Autodesk Inventor part; units mm, degrees
ref_plane "YZ Plane" through (0, 0, 0) normal (1, 0, 0) x (0, 1, 0)
ref_plane "XZ Plane" through (0, 0, 0) normal (0, 1, 0) x (-1, 0, 0)
ref_plane "XY Plane" through (0, 0, 0) normal (0, 0, 1) x (1, 0, 0)
sketch "Sketch1" plane through (0, 0, 0) normal (1, 0, 0) x (0, 1, 0)
  line L0 (31.75, 38.1) -> (6.35, 38.1)
  line L1 (6.35, 38.1) -> (6.35, -19.05)
  line L2 (6.35, -19.05) -> (31.75, -19.05)
  circle A0 centre (19.0246, 25.4) radius 3.175
  line L3 (0, 0) -> (6.35, 0)
  line L4 (0, 14.2875) -> (0, -6.35)
  circle A1 centre (19.05, -7.62) radius 3.175
  line L5 (31.75, 38.1) -> (31.75, -25.4)
  point P0 (31.75, -19.05)
  dimension "d0" = 57.15
  dimension "d1" = 38.1
  dimension "d2" = 25.4
  dimension "d3" = 31.75
  dimension "d4" = 6.35
  dimension "d7" = 6.35
  dimension "d8" = 33.02
extrude "Extrusion1" add sketch "Sketch1" along normal blind 25.4
sketch "Sketch2" plane through (0, 6.35, 38.1) normal (0, 0, 1) x (1, 0, 0)
  line L0 (0, 25.4) -> (25.4, 25.4)
  line L1 (25.4, 0) -> (0, 0)
  line L2 (0, 0) -> (0, 25.4)
  line L3 (0, 25.4) -> (25.4, 25.4)
  line L4 (25.4, 25.4) -> (25.4, 0)
  point P0 (0, -6.35)
extrude "Extrusion2" add sketch "Sketch2" along normal blind 25.4
sketch "Sketch3" plane through (0, 6.35, 63.5) normal (0, 0, 1) x (1, 0, 0)
  circle A0 centre (12.7, 12.7) radius 6.35
  point P0 (0, -6.35)
  dimension "d18" = 12.7
extrude "Extrusion3" add sketch "Sketch3" along normal blind 88.9
properties part number "Base"
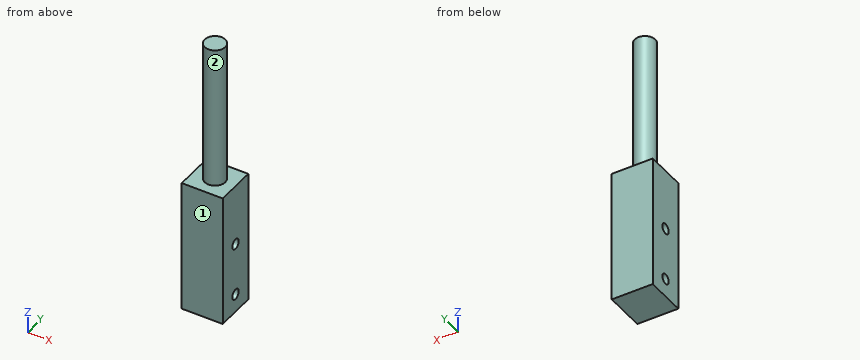
Geometry check sheet. Reference: the model listing, model coordinates, mm. Face numbers are marked on the shaded views. A direction names the side the tool comes from. Give positions to 0.01 mm unless a question says otherwise; leave off trailing zeros. Order: outer loops, then holes, each group sorted by start corner. A loop starts at its lowest first (then second) coordinate and runs counter-clockwise, first axis right, second up.
1. Section check B-B, the plane x = 12.7. Enter the section's corners in (y, z) (3 decimals).
2. Thickness scan on L1, parallel to Z at x = 7, y = 19.05 (3 decimals); L2, parallel to Z at x = 13, y = 21.5; L3, parallel to X at y = 18.5, z = 127.5. Record the ranges inside material, lowest first.
3. Section check A-A, the plane z = 25.4. Enter the section's corners in (x, y), and give its area (3 significant figures).
4. Access from +Z, -Z, +X, -X, +Y, -Y to the whole of each face (thin tool, end or side, straight path). Record for the marked faces 1 and 2.
5. Section check D-D, the plane y = 11.25. Enter the section's corners in (x, z).
6. Gauge pin test, flat ends, axial feed: pin 1 Ø1.5 at (y, z) = (24, 110) entering from -X; pin 2 Ø1 at (x, y) = (7, 27.5) entering from +Z; pin 3 Ø8 at (y, z) = (15, 134.5) entering from +X; pin 4 Ø1 at (y, z) = (10.5, 111.5) entering from -X. Record the tip position at first contact, or that the pin passes through.
7. Section check C-C, the plane y = 19.05. Enter the section's corners in (x, z) (3 decimals).
Values follow:
1. outline: (6.35, -19.05) - (31.75, -19.05) - (31.75, 63.5) - (25.4, 63.5) - (25.4, 152.4) - (12.7, 152.4) - (12.7, 63.5) - (6.35, 63.5) - close; hole circle Ø6.35 at (19.025, 25.4); hole circle Ø6.35 at (19.05, -7.62)
2. L1: z = -19.05 to -10.795, -4.445 to 22.225, 28.575 to 152.4
2. L2: z = -19.05 to -9.64, -5.6 to 23.41, 27.39 to 152.4
2. L3: x = 6.37 to 19.03
3. outline: (0, 6.35) - (25.4, 6.35) - (25.4, 15.85) - (0, 15.85) - close; (0, 22.2) - (25.4, 22.2) - (25.4, 31.75) - (0, 31.75) - close
3. area: 484 mm2
4. face 1: +Z, -Z, +X, -X, -Y
4. face 2: +Z
5. outline: (0, -19.05) - (25.4, -19.05) - (25.4, 63.5) - (0, 63.5) - close
6. pin 1: stops at x = 7.94
6. pin 2: stops at z = 63.5
6. pin 3: stops at x = 19.05
6. pin 4: passes through
7. outline: (0, -19.05) - (25.4, -19.05) - (25.4, -10.795) - (0, -10.795) - close; (0, -4.445) - (25.4, -4.445) - (25.4, 22.225) - (0, 22.225) - close; (0, 28.575) - (25.4, 28.575) - (25.4, 63.5) - (19.05, 63.5) - (19.05, 152.4) - (6.35, 152.4) - (6.35, 63.5) - (0, 63.5) - close
